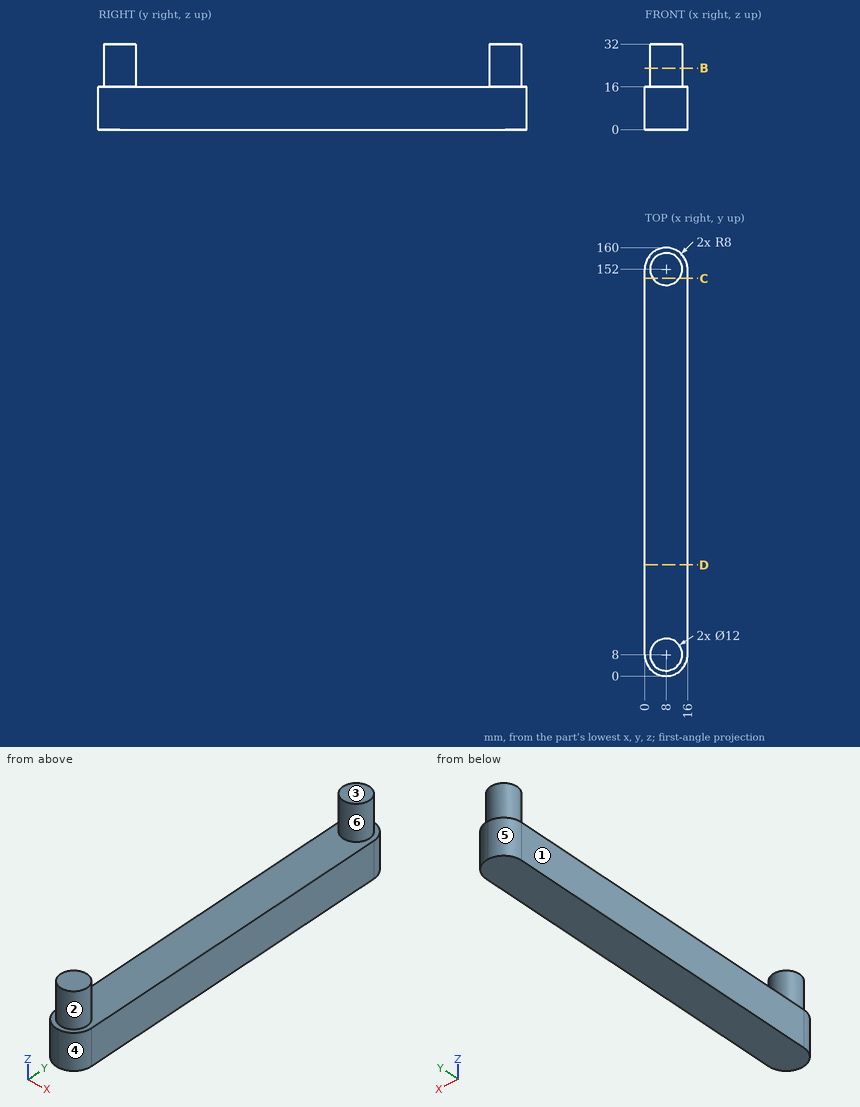
Here's the drawing with two shaded views (mm, measured from the low corner). I have some questions. A direction names the side the tool comes from. Round coordinates to 2 decimals unless told otherwise and drop trailing zeros. Write each loop counter-clockwise with the first axis right and the second up, starting at its lowest first coordinate (ties: lowest second). Pieces come first, ordered by that corner, then holes. Notation, with made-up numbers: M 4.25,-36 L 40.25,-36 A20 cw 40.25,-11 Z; hole C 27.25,63.5 d7. An arc over 180 degrees is marked long. Write each question's results on one line, items separated by ' | '. Start each with the question number.
1. I'm going to push flat-ended pins straight in: pin 1 Ø1.5 at (x, z) = (8, 27) entering from -Y; pin 2 Ø3 at (x, z) = (11, 23.5) entering from +Y; pin 3 Ø5 at (x, y) = (6.5, 85) entering from +Z. Where does each tip first touch, or does it pass through?
2. Thinking about a two-plate mould opening in Y: for the marked faces 3, 4, 5 and 6, which applies, +Y half, -Y half, draft (parallel to the pull), parting line (faces both ways), or undercut?
3. Imagine slicing it at B-B on z = 23. List the corners of the cut face in (x, y) for me, and give its area (3 significant figures).
4. I need wall thicknesses on L1, parallel to Y at x = 8.5, z = 26; L2, parallel to Y at x = 3.75, z = 18.5 (1 decimal); L3, parallel to Z at x = 2.75, y = 118. Which ranges of each line are inside material? Lowest first, please. Write a range as from..to.
5. Imagine slicing it at C-C on y = 148.5. List the corners of the cut face in (x, z) for me, and give its area (3 significant figures).
6. On a 3-axis mill with a long thin cutter (end or side, diameter ignored), from which of +Z, -Z, +X, -X, +Y, -Y can I reach the whole of each face in a straight line? I mean the marked faces 1 and 2. Say none if no direction works.
7. Imagine slicing it at D-D on y = 41.5. List the corners of the cut face in (x, z) for me, and give its area (3 significant figures).
Result sheet:
1) pin 1: stops at y = 2 | pin 2: stops at y = 157.81 | pin 3: stops at z = 16
2) face 3: draft | face 4: -Y half | face 5: +Y half | face 6: undercut
3) outline: C 8,8 d12; C 8,152 d12 | area: 226 mm^2
4) L1: y = 2.02..13.98, 146.02..157.98 | L2: y = 3.8..12.2, 147.8..156.2 | L3: z = 0..16
5) outline: M 0,0 L 16,0 L 16,16 L 12.87,16 L 12.87,32 L 3.13,32 L 3.13,16 L 0,16 Z | area: 412 mm^2
6) face 1: +Z, -Z, -X, +Y, -Y | face 2: +Z
7) outline: M 0,0 L 16,0 L 16,16 L 0,16 Z | area: 256 mm^2
